Input: part model. Units: mm. Frame: model coordinates. Round coordinates to 2 decimals unless told otherwise and drop trailing zeros. Use a Markdown table: item, result.
from build123d import *

# Parameters (mm, degrees)
SKETCH1_R                = 5
BOSS_EXTRUDE1_DEPTH      = 2.54
F_3_0_3_DIAMETER_HOLE1_D = 3


with BuildPart() as part:
    # Sketch1 → Boss-Extrude1 (new body)
    with BuildSketch(Plane(origin=(0, 0, 0), x_dir=(1, 0, 0), z_dir=(0, 1, 0))):
        Polygon((-107.5, -77.5), (-107.5, -120), (107.5, -120), (107.5, -77.5), (120, -77.5), (120, 120), (-120, 120), (-120, -77.5), align=None)
        with Locations(Location((-22.5, -10, 0), (0, 0, 270))):
            Circle(SKETCH1_R, mode=Mode.SUBTRACT)
    extrude(amount=BOSS_EXTRUDE1_DEPTH)

    # Ø3.0 (3) Diameter Hole1 (through all)
    with Locations(Plane.XZ):
        with Locations((-103.5, 116), (-62.1, 116), (-20.7, 116), (20.7, 116), (62.1, 116), (103.5, 116), (116, 73.5), (116, 49), (116, 14), (116, -36), (116, -70), (105, -116), (63, -116), (21, -116), (-21, -116), (-63, -116), (-105, -116), (-116, -59), (-116, -24), (-116, 26), (-116, 69.5)):
            Hole(F_3_0_3_DIAMETER_HOLE1_D / 2)


solid = part.part
1) Pull-direction query (Z, two-part tool) for faces 1 (the cylindrical face through (-26.936, 1.252, 12.307)), 2 (the flat face through (-2, 2.54, -2)); classes: +Z half, -Z half, draft (parallel to the pull), parting line (faces both ways), or undercut.
Results found:
| item | result |
|---|---|
| face 1 | undercut |
| face 2 | draft |
2) Line query: L1, parallel to Z at x = -116, y = 1.6; L2, parallel to Z at x = 21, y = 0.7; L3, parallel to Z at x = 63, y = 1.35. Output: solid intervals per line, ascending. Write a range as [from, to].
Results found:
| item | result |
|---|---|
| L1 | z = [-120, -60.5], [-57.5, -25.5], [-22.5, 24.5], [27.5, 68], [71, 77.5] |
| L2 | z = [-120, -117.5], [-114.5, 114.53], [117.47, 120] |
| L3 | z = [-120, -117.5], [-114.5, 114.8], [117.2, 120] |
3) Pin query (flat end, axial travel): pin 1 Ø2.5 at (x, z) = (103.5, 116) entering from -Y; pin 2 Ø1.3 at (x, y) = (-111, 2) entering from +Z. Return the tip coordinate at first contact, or that it passes through.
Results found:
| item | result |
|---|---|
| pin 1 | passes through |
| pin 2 | stops at z = 77.5 |
4) Cut plane A-A on y = 1.6. Count the separate pieces of the cut face and the enclosed holes in it, and give its area (3 significant figures).
Results found:
| item | result |
|---|---|
| separate pieces | 1 |
| enclosed holes | 22 |
| area | 56,300 mm² |
